```python
from build123d import *

# Parameters (mm, degrees)
EXTRUDE_1_DEPTH     = 5
SKETCH_2_R          = 18
EXTRUDE_2_DEPTH     = 35
EXTRUDE_START       = 20
SKETCH_3_R          = 18
EXTRUDE_3_DEPTH     = 20
SKETCH_4_R          = 15
CUT_EXTRUDE_1_DEPTH = 55
SKETCH_5_R          = 6
SKETCH_5_R_2        = 4
EXTRUDE_4_DEPTH     = 5
CUT_EXTRUDE_2_REACH = 103.119
SKETCH_6_R          = 4
FILLET_1_R          = 5


with BuildPart() as part:
    # 草图1 → 凸台-拉伸1 (new body)
    with BuildSketch(Plane.XY):
        with BuildLine():
            Line((-20.712315177, 14), (-41, 14))
            Line((-41, 14), (-59, 30))
            Line((-59, 30), (-90, 30))
            Line((-90, 30), (-90, 15))
            Line((-90, 15), (-85, 15))
            Line((-85, 15), (-85, -15))
            Line((-85, -15), (-90, -15))
            Line((-90, -15), (-90, -30))
            Line((-90, -30), (-59, -30))
            Line((-59, -30), (-41, -14))
            Line((-41, -14), (-20.712315177, -14))
            ThreePointArc((-20.712315177, -14), (0, -25), (20.712315177, -14))
            Line((20.712315177, -14), (41, -14))
            Line((41, -14), (59, -30))
            Line((59, -30), (90, -30))
            Line((90, -30), (90, -15))
            Line((90, -15), (85, -15))
            Line((85, -15), (85, 15))
            Line((85, 15), (90, 15))
            Line((90, 15), (90, 30))
            Line((90, 30), (59, 30))
            Line((59, 30), (41, 14))
            Line((41, 14), (20.712315177, 14))
            ThreePointArc((20.712315177, 14), (0, 25), (-20.712315177, 14))
        make_face()
    extrude(amount=EXTRUDE_1_DEPTH)

    # 草图2 → 凸台-拉伸2 (add)
    with BuildSketch(Plane.XY.offset(5)):
        Circle(SKETCH_2_R)
    extrude(amount=EXTRUDE_2_DEPTH)

    # 草图3 → 凸台-拉伸3 (add)
    with BuildSketch(Plane(origin=(0, 0, 0), x_dir=(-1, 0, 0), z_dir=(0, 0, -1)).offset(EXTRUDE_START)):
        with Locations(Location((0, 0, 0), (0, 0, 180))):
            Circle(SKETCH_3_R)
    extrude(amount=-EXTRUDE_3_DEPTH)

    # 草图4 → 切除-拉伸1 (cut)
    with BuildSketch(Plane(origin=(0, 0, -20), x_dir=(-1, 0, 0), z_dir=(0, 0, -1))):
        Circle(SKETCH_4_R)
    extrude(amount=-CUT_EXTRUDE_1_DEPTH, mode=Mode.SUBTRACT)

    # 草图5 → 凸台-拉伸4 (add)
    # profile 1 of 2: a face of its own
    with BuildSketch(Plane.XY.offset(5)):
        with Locations((-31, 0)):
            Circle(SKETCH_5_R)
        with Locations((-31, 0)):
            Circle(SKETCH_5_R_2, mode=Mode.SUBTRACT)
    # profile 2 of 2: a face of its own
    with BuildSketch(Plane.XY.offset(5)):
        with Locations((31, 0)):
            Circle(SKETCH_5_R)
        with Locations((31, 0)):
            Circle(SKETCH_5_R_2, mode=Mode.SUBTRACT)
    extrude(amount=EXTRUDE_4_DEPTH)

    # 草图6 → 切除-拉伸2 (cut, up to next)
    with BuildSketch(Plane.XY.offset(5), mode=Mode.PRIVATE) as cut_extrude_2_sk1:
        with Locations((31, 0)):
            Circle(SKETCH_6_R)
    cut_extrude_2_tool1 = extrude(cut_extrude_2_sk1.sketch, amount=-CUT_EXTRUDE_2_REACH, mode=Mode.PRIVATE) & part.part
    # 草图6 → 切除-拉伸2 (cut, up to next)
    with BuildSketch(Plane.XY.offset(5), mode=Mode.PRIVATE) as cut_extrude_2_sk2:
        with Locations((-31, 0)):
            Circle(SKETCH_6_R)
    cut_extrude_2_tool2 = extrude(cut_extrude_2_sk2.sketch, amount=-CUT_EXTRUDE_2_REACH, mode=Mode.PRIVATE) & part.part
    add(cut_extrude_2_tool1.solids().sort_by_distance((31, 0, 5))[0], mode=Mode.SUBTRACT)
    add(cut_extrude_2_tool2.solids().sort_by_distance((-31, 0, 5))[0], mode=Mode.SUBTRACT)

    # 圆角1
    fillet_1_edges = [part.edges().sort_by_distance(p)[0] for p in [
        (90, 30, 2.5),
        (90, -30, 2.5),
        (-90, -30, 2.5),
        (-90, 30, 2.5),
    ]]
    fillet(fillet_1_edges, radius=FILLET_1_R)


solid = part.part
```
Check sheet for the modelled part. Datum: model origin and axes. Units: mm. A direction names the side the tool comes from. Coordinates: 2 decimals unless noted, no trailing zeros. Loops run counter-clockwise (first coordinate to the right, second up) from the corner with the lowest first, then second, coordinate; pieces in that order, holes last.
1) Release check for a two-part mould opening along X. For faces 4 (the face through (14.985, 0.66, 7.115)), 5 (the face through (90, -20, 2)), 6 (the face through (34.92, 1.42, 10)) record: released by +X, released by -X, zero draft, split by the parting line, or undercut.
2) Access from +Z, -Z, +X, -X, +Y, -Y to the whole of each face (thin tool, end or side, straight path). Record for faces 1 (the face through (50, -22, 2)), 2 (the face through (-85, 0, 2)), 3 (the face through (88, -15, 2)).
3) Sectioned sample at D-D (z = -6). Record the boundary of the cut face in (x, y), and give its area (3 significant figures).
4) Sectioned sample at B-B (x = -31). Record the boundary of the cut face in (y, z), and give its area (3 significant figures).
5) Material ranges on probe 1 along Y at (x, z) = (-31, 7); probe 2 along Z at (x, y) = (65, -13.5); probe 3 along X at (y, z) = (-8, 32.5), recorded low to high.
6) Gauge pin test, flat ends, axial feed: pin 1 (5.5 mm diameter, centred on x = 28.5, z = 1.5, fed in from -Y); pin 2 (1.5 mm diameter, centred on x = 88.5, z = 3.5, fed in from +Y); pin 3 (2 mm diameter, centred on x = -1.5, z = 28, fed in from +Y). Record the tip position at first contact, or that the pin passes through.
7) Sectioned sample at C-C (x = 0). Record the boundary of the cut face in (y, z).
8) Sectioned sample at A-A (y = 0). Count the separate pieces of the cut face and the enclosed holes in it, and give its area (3 significant figures).
Check sheet entries:
1. face 4: undercut
1. face 5: released by +X
1. face 6: zero draft
2. face 1: +Z, -Z, -Y
2. face 2: +Z, -Z, -X
2. face 3: +Z, -Z, +X
3. outline: circle Ø36 at (0, 0); hole circle Ø30 at (0, 0)
3. area: 311 mm2
4. outline: (-14, 0) - (-4, 0) - (-4, 10) - (-6, 10) - (-6, 5) - (-14, 5) - close; (4, 0) - (14, 0) - (14, 5) - (6, 5) - (6, 10) - (4, 10) - close
4. area: 120 mm2
5. probe 1: y = -6 to -4, 4 to 6
5. probe 2: z = 0 to 5
5. probe 3: x = -16.12 to -12.69, 12.69 to 16.12
6. pin 1: stops at y = -14
6. pin 2: stops at y = 29.18
6. pin 3: stops at y = 17.99
7. outline: (-25, 0) - (-18, 0) - (-18, -20) - (-15, -20) - (-15, 35) - (15, 35) - (15, -20) - (18, -20) - (18, 0) - (25, 0) - (25, 5) - (18, 5) - (18, 40) - (-18, 40) - (-18, 5) - (-25, 5) - close
8. separate pieces: 3
8. enclosed holes: 0
8. area: 1,140 mm2
